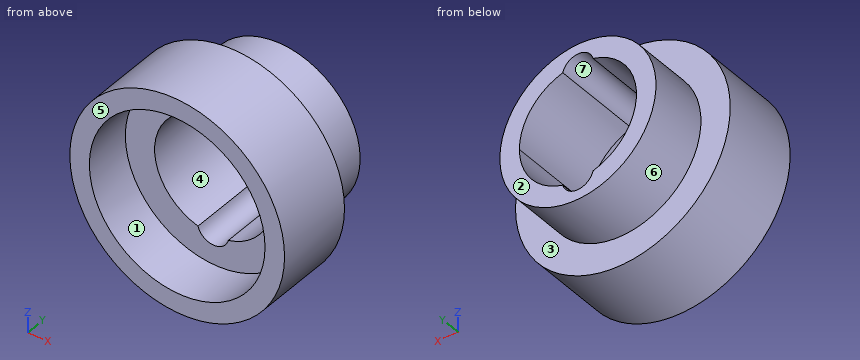
```python
from build123d import *

# Parameters (mm, degrees)
F0_R     = 20
F1_DEPTH = 35
F2_R     = 27.5
F2_R_2   = 20
F3_DEPTH = 20
F4_R     = 22.5
F5_DEPTH = 12


with BuildPart() as f1:
    # F0 (on Front) → F1 (new body)
    with BuildSketch(Plane.XZ):
        Circle(F0_R)
        with BuildLine():
            ThreePointArc((3.875362, 14.490741), (11.898118, 9.134264), (15, 0))
            ThreePointArc((15, 0), (11.898118, -9.134264), (3.875362, -14.490741))
            ThreePointArc((3.875362, -14.490741), (0, -17.5), (-3.875362, -14.490741))
            ThreePointArc((-3.875362, -14.490741), (-15, 0), (-3.875362, 14.490741))
            ThreePointArc((-3.875362, 14.490741), (0, 17.5), (3.875362, 14.490741))
        make_face(mode=Mode.SUBTRACT)
    extrude(amount=F1_DEPTH)

    # F2 (on face) → F3 (join)
    with BuildSketch(Plane.XZ.offset(35)):
        Circle(F2_R)
        Circle(F2_R_2, mode=Mode.SUBTRACT)
    extrude(amount=-F3_DEPTH)

    # F4 (on face) → F5 (cut)
    with BuildSketch(Plane.XZ.offset(35)):
        Circle(F4_R)
    extrude(amount=-F5_DEPTH, mode=Mode.SUBTRACT)


solid = f1.part
```
Could you check a few things on this model? Use its own coordinates, in mm. Face numbers are marked on the shaded views. A direction names the side the tool comes from. Coordinates: 2 decimals unless noted, no trailing zeros. Order: outer loops, then holes, each group sorted by start corner. A loop starts at its lowest first (then second) coordinate and runs counter-clockwise, first axis right, second up. Notation, with made-up numbers: M -0.75,70.5 L 25.25,70.5 A31 ccw 25.25,99.5 Z; hole C 19.5,-8 d3. An arc over 180 degrees is marked long. Use a Markdown table: item, result. Add a question column.
Q1. Which directions (+Z, -Z, +X, -X, +Y, -Y) give clear straight access to the entire face, cutting with the end or side of a thin tool? Please do the marked faces 1, 2, 3 and 4.
Q2. I want a section at D-D on y = -26. List the corners of the cut face in (x, z) for me.
Q3. I want a section at B-B on x = -1. List the corners of the cut face in (y, z) for me.
Q4. If I drill on L1, parallel to Y at x = 17, z = -1; L2, parallel to Y at x = -18.5, z = 11; L3, parallel to X at y = -25.5, z = 19.5, over which ranges is the centre line in solid material (lowest first)?
Q5. We'd pull the mould along X, two halves only. Please class the marked faces 5, 6 and 7: pulls with the +X half, pulls with the -X half, needs draft (parallel to the pull), parting line crosses it, or undercut.
Q6. I'm going to push flat-ended pins straight in: pin 1 (8 mm diameter, centred on y = -11.5, z = 10.5, fed in from -X); pin 2 (10 mm diameter, centred on x = -19.5, y = -27, fed in from +Z); pin 3 (5 mm diameter, centred on x = -8, z = 14.5, fed in from +Y); pin 4 (6 mm diameter, centred on y = -29.5, z = 3.5, fed in from -X). Where does each tip first touch, or does it pass through?
Q7. I want a section at A-A on z = -5. List the corners of the cut face in (x, y) for me, then the cut area to 3 significant figures.
Q8. I want a section at C-C on y = -8. List the corners of the cut face in (x, z) for me, then the cut area to 3 significant figures.
Checked values:
| question | item | result |
|---|---|---|
| 1 | face 1 | -Y |
| 1 | face 2 | +Z, -Z, +X, -X, +Y |
| 1 | face 3 | +Y |
| 1 | face 4 | +Y, -Y |
| 2 | outline | C 0,0 d55; hole C 0,0 d45 |
| 3 | outline | M -35,-27.48 L -15,-27.48 L -15,-19.97 L 0,-19.97 L 0,-17.37 L -23,-17.37 L -23,-22.48 L -35,-22.48 Z; M -35,22.48 L -23,22.48 L -23,17.37 L 0,17.37 L 0,19.97 L -15,19.97 L -15,27.48 L -35,27.48 Z |
| 4 | L1 | -23 to 0 |
| 4 | L2 | -23 to -15 |
| 4 | L3 | -19.39 to -11.22, 11.22 to 19.39 |
| 5 | face 5 | needs draft |
| 5 | face 6 | parting line crosses it |
| 5 | face 7 | undercut |
| 6 | pin 1 | x = -26.13 |
| 6 | pin 2 | z = 23.37 |
| 6 | pin 3 | y = 0 |
| 6 | pin 4 | x = -27.5 |
| 7 | outline | M -27.04,-35 L -21.94,-35 L -21.94,-23 L -14.14,-23 L -14.14,0 L -19.36,0 L -19.36,-15 L -27.04,-15 Z; M 14.14,-23 L 21.94,-23 L 21.94,-35 L 27.04,-35 L 27.04,-15 L 19.36,-15 L 19.36,0 L 14.14,0 Z |
| 7 | area | 486 mm² |
| 8 | outline | C 0,0 d40; hole M -3.88,-14.49 A4 ccw 3.88,-14.49 A15 ccw 15,0 A15 ccw 3.88,14.49 A4 ccw -3.88,14.49 A15 ccw Z |
| 8 | area | 520 mm² |
